Check sheet for the drawn part. Datum: minimum x, y, z corner. Units: mm. A direction names the side the tool comes from. Coordinates: 2 decimals unless noted, no trailing zeros. Order: outer loops, then holes, each group sorted by start corner. A loop starts at its lowest first (then second) coordinate and runs counter-clockwise, first axis right, second up.
1. Cross-section at D-D (z = 32). Enter the section's corners in (x, y) (1 decimal), then the cut area to 3 significant figures.
2. Draft check along Y on the marked faces 4, 5 and 6. Enter one of: released by +Y, released by -Y, zero draft, split by the parting line, or undercut.
3. Set-up check for the marked faces 1, 2 and 3: record each of +Z, -Z, +X, -X, +Y, -Y from which the full face is reachable in a straight line by a thin tool's end or side.
4. Cross-section at B-B (x = 11.5). Enter the section's corners in (y, z).
5. Cross-section at C-C (y = 46). Enter the section's corners in (x, z), then the cut area to 3 significant figures.
6. Gauge pin test, flat ends, axial feed: pin 1 Ø3 at (x, z) = (47, 20.5) entering from +Y; pin 2 Ø3 at (x, y) = (57, 62) entering from -Z; pin 3 Ø6 at (x, y) = (63.99, 36.07) entering from +Z. Record the tip position at first contact, or that the pin passes through.
7. Cross-section at A-A (z = 38). Enter the section's corners in (x, y) (1 decimal), then the cut area to 3 significant figures.
8. Thickness scan on line 1 (X direction, y = 38, z = 35) (1 decimal); line 2 (Y direction, x = 6.5, z = 29) (1 decimal); line 3 (Y direction, x = 7.5, z = 29.5) (1 decimal). Record the ranges inside material, lowest first.
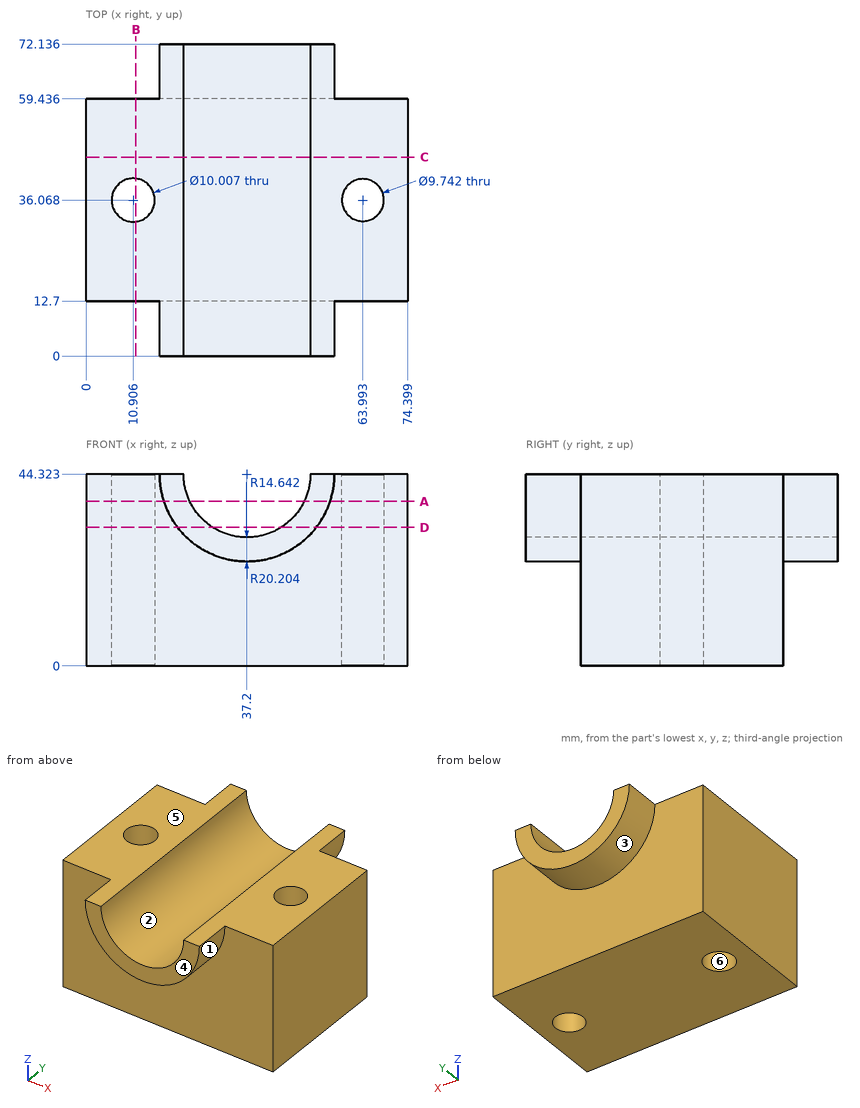
Data:
1. outline: (0, 12.7) - (21.2, 12.7) - (21.2, 0) - (29.3, 0) - (29.3, 72.1) - (21.2, 72.1) - (21.2, 59.4) - (0, 59.4) - close; (45.1, 0) - (53.2, 0) - (53.2, 12.7) - (74.4, 12.7) - (74.4, 59.4) - (53.2, 59.4) - (53.2, 72.1) - (45.1, 72.1) - close; hole circle Ø10 at (10.9, 36.1); hole circle Ø9.7 at (64, 36.1)
1. area: 3,000 mm2
2. face 4: released by -Y
2. face 5: zero draft
2. face 6: undercut
3. face 1: -Z, -Y
3. face 2: +Z, +Y, -Y
3. face 3: -Z, +Y
4. outline: (12.7, 0) - (31.1, 0) - (31.1, 44.32) - (12.7, 44.32) - close; (41.04, 0) - (59.44, 0) - (59.44, 44.32) - (41.04, 44.32) - close
5. outline: (0, 0) - (74.4, 0) - (74.4, 44.32) - (51.84, 44.32) arc R14.64 cw to (22.56, 44.32) - (0, 44.32) - close
5. area: 2,960 mm2
6. pin 1: stops at y = 59.44
6. pin 2: stops at z = 35.76
6. pin 3: passes through
7. outline: (0, 12.7) - (18, 12.7) - (18, 0) - (24, 0) - (24, 72.1) - (18, 72.1) - (18, 59.4) - (0, 59.4) - close; (50.4, 0) - (56.4, 0) - (56.4, 12.7) - (74.4, 12.7) - (74.4, 59.4) - (56.4, 59.4) - (56.4, 72.1) - (50.4, 72.1) - close; hole circle Ø10 at (10.9, 36.1); hole circle Ø9.7 at (64, 36.1)
7. area: 2,390 mm2
8. line 1: x = 0 to 6.3, 15.5 to 25.9, 48.5 to 59.5, 68.5 to 74.4
8. line 2: y = 12.7 to 33.7, 38.4 to 59.4
8. line 3: y = 12.7 to 32.4, 39.7 to 59.4
